Input: part model. Units: mm. Frame: model coordinates. A direction names the side the tool comes from. Round coordinates to 2 decimals unless told otherwise and drop trailing zeros. Write each loop counter-clockwise with the first axis right and the second up, starting at its lowest first coordinate (ties: lowest second). Pieces come first, ordered by that corner, then holes. Notation, with made-up numbers: (18.25, -14.75) -> (55.25, -14.75) arc R24 ccw to (55.25, 10.25) -> close; hole circle Ø4 at (82, -33.5). An arc over 180 degrees is marked (long way). Use CSV: the item, a comma, the result in double quotes.
Autodesk Fusion 360 part; units mm, degrees
sketch "Sketch1" plane through (0, 0, 0) normal (0, 1, 0) x (1, 0, 0)
  line L0 (-18, 25) -> (0, 25)
  line L1 (-50.0002, -10) -> (-50, 12)
  line L2 (-50, 12) -> (-18, 12)
  line L3 (-18, 12) -> (-18, 25)
  line L4 (-50.0002, -10) -> (-10, -10)
  line L5 (0, 0) -> (0, 25)
  arc A0 (-10, -10) -> (0, 0) centre (-10, 0) ccw
  dimension "d6" = 18
  dimension "d7" = 50
  dimension "d8" = 13
  dimension "d10" = 22
  dimension "d11" = 10
extrude "Extrude1" add sketch "Sketch1" along normal mid plane 55
sketch "Sketch2" plane through (0, 0, 10) normal (0, 0, 1) x (-1, 0, 0)
  line L0 (10, 27.5) -> (10, -27.5)
  line L1 (10, -27.5) -> (50.0002, -27.5)
  line L2 (50.0002, -27.5) -> (50.0002, 27.5)
  line L3 (50.0002, 27.5) -> (10, 27.5)
  circle A0 centre (30.0002, 12.5) radius 7
  circle A1 centre (30.0002, -12.5) radius 7
  dimension "d17" = 14
  dimension "d18" = 15
  dimension "d19" = 20
  dimension "d20" = 14
  dimension "d21" = 15
  dimension "d22" = 20
extrude "Extrude2" cut sketch "Sketch2" against normal through all contours A0 | A1
sketch "Sketch3" plane through (0, 0, 0) normal (0, 1, 0) x (1, 0, 0)
  line L0 (-50, 2) -> (-112, 2)
  line L1 (-50, -10) -> (-90, -10)
  line L2 (-112, 2) -> (-112, -50)
  line L3 (-90, -10) -> (-90, -70)
  line L4 (-90, -70) -> (-165, -70)
  line L5 (-165, -70) -> (-165, -50)
  line L6 (-165, -50) -> (-112, -50)
  line L7 (-50, -10) -> (-50, 2)
  dimension "d24" = 62
  dimension "d26" = 40
  dimension "d28" = 52
  dimension "d30" = 75
  dimension "d31" = 20
  dimension "d52" = 12
extrude "Extrude3" add sketch "Sketch3" along normal mid plane 15
fillet "Fillet1" radius 6 1 edges at (-112, 0, -2)
sketch "Sketch5" plane through (0, -7.5, 0) normal (0, -1, 0) x (1, 0, 0)
  arc A0 (-112, 4) -> (-106, -2) centre (-106, 4) ccw
  line L0 (-106, -2) -> (-50.0001, -2)
  line L1 (-50.0001, -2) -> (-50.0002, 10)
  line L2 (-50.0002, 10) -> (-90, 10)
  line L3 (-90, 10) -> (-90, 70)
  line L4 (-90, 70) -> (-165, 70)
  line L5 (-165, 70) -> (-165, 50)
  line L6 (-165, 50) -> (-112, 50)
  line L7 (-112, 50) -> (-112, 4)
  line L8 (-115, 63) -> (-165, 63)
  line L9 (-165, 63) -> (-165, 88)
  line L10 (-165, 88) -> (-150, 88)
  line L11 (-150, 88) -> (-150, 73)
  line L12 (-150, 73) -> (-130, 73)
  line L13 (-130, 73) -> (-130, 88)
  line L14 (-130, 88) -> (-115, 88)
  line L15 (-115, 88) -> (-115, 63)
  dimension "d41" = 50
  dimension "d42" = 25
  dimension "d43" = 15
  dimension "d44" = 15
  dimension "d45" = 20
  dimension "d46" = 15
  dimension "d47" = 18
extrude "Extrude4" add sketch "Sketch5" along normal blind 15 and the other way blind 40 contours L4 L5 L8 L9 L15 | L4 L9 L10 L11 L12 L13 L14 L15
sketch "Sketch6" plane through (0, -7.5, 0) normal (0, -1, 0) x (1, 0, 0)
  line L0 (-115, 63) -> (-165, 63)
  line L1 (-165, 63) -> (-165, 50)
  line L2 (-165, 50) -> (-112, 50)
  line L3 (-112, 50) -> (-112, 4)
  arc A0 (-112, 4) -> (-106, -2) centre (-106, 4) ccw
  line L4 (-106, -2) -> (-50.0001, -2)
  line L5 (-50.0001, -2) -> (-50.0002, 10)
  line L6 (-50.0002, 10) -> (-90, 10)
  line L7 (-90, 10) -> (-90, 70)
  line L8 (-90, 70) -> (-115, 70)
  line L9 (-115, 70) -> (-115, 63)
sketch "Sketch7" plane through (0, -7.5, 0) normal (0, -1, 0) x (1, 0, 0)
Item 1: Section query D-D on y = 2.5. Return the cut outline in (x, z).
Worked answers:
outline,"(-165, 50) -> (-112, 50) -> (-112, 4) arc R6 ccw to (-106, -2) -> (-50, -2) -> (-50, -12) -> (-18, -12) -> (-18, -25) -> (0, -25) -> (0, 0) arc R10 ccw to (-10, 10) -> (-90, 10) -> (-90, 70) -> (-115, 70) -> (-115, 88) -> (-130, 88) -> (-130, 73) -> (-150, 73) -> (-150, 88) -> (-165, 88) -> close"
Item 2: First-contact query: pin 1 Ø12.5 at (y, z) = (13.5, 81.5) entering from +X; pin 2 Ø11 at (x, y) = (-30, -12.5) entering from +Z (3 decimals); pin 3 Ø10 at (y, z) = (-8, 28) entering from +X; pin 4 Ø12 at (x, y) = (-145.5, -18.5) entering from -Z. Flat tips, straight axial feed; report the tip coordinate or a pass-through.
Worked answers:
pin 1,"stops at x = -115"
pin 2,"passes through"
pin 3,"stops at x = -90"
pin 4,"stops at z = 63"
Item 3: Set-up query: faces 4 (the face through (-140, -15, 63)), 5 (the face through (-130, 5, 80)), 6 (the face through (-112, 0, 27)). Return all of +Z, -Z, +X, -X, +Y, -Y with unobstructed straight access to the full face (end or side cutting, diameter ignored); none if empty.
Worked answers:
face 4,"-Z, +X, -X, -Y"
face 5,"+Z, +Y, -Y"
face 6,"-Z, -X, +Y, -Y"
Item 4: Section query A-A on y = -12.5. Return the cut outline in (x, z), plus the area to 3 significant figures.
Worked answers:
outline,"(-165, 63) -> (-115, 63) -> (-115, 88) -> (-130, 88) -> (-130, 73) -> (-150, 73) -> (-150, 88) -> (-165, 88) -> close; (-50, -12) -> (-37, -12) -> (-37, 10) -> (-50, 10) -> close; (-23, -12) -> (-18, -12) -> (-18, -25) -> (0, -25) -> (0, 0) arc R10 ccw to (-10, 10) -> (-23, 10) -> close"
area,"1,950 mm²"
Item 5: Section query B-B on z = 68. Return the cut outline in (x, y).
Worked answers:
outline,"(-165, -22.5) -> (-115, -22.5) -> (-115, -7.5) -> (-90, -7.5) -> (-90, 7.5) -> (-115, 7.5) -> (-115, 32.5) -> (-165, 32.5) -> close"
Item 6: Line query: line 1 (X direction, y = 6.5, z = 77.5); line 2 (X direction, y = -12.5, z = -4); line 3 (Z direction, x = -51.5, y = -4). Output: solid intervals per line, ascending.
Worked answers:
line 1,"x = -165 to -150, -130 to -115"
line 2,"x = -50 to -37, -23 to 0"
line 3,"z = -2 to 10"
Item 7: Pull-direction query (X, two-part tool) for faces 1 (the face through (-18, 0, -18)), 2 (the face through (-150, 5, 81)), 3 (the face through (-78, 0, -2)); classes: +X half, -X half, draft (parallel to the pull), parting line (faces both ways), or undercut.
Worked answers:
face 1,"-X half"
face 2,"undercut"
face 3,"draft"
Item 8: Section query C-C on x = -153.5. Return the cut outline in (y, z), plus the area to 3 significant figures.
Worked answers:
outline,"(-22.5, 63) -> (-7.5, 63) -> (-7.5, 50) -> (7.5, 50) -> (7.5, 63) -> (32.5, 63) -> (32.5, 88) -> (-22.5, 88) -> close"
area,"1,570 mm²"
